Build history of the part. All positions in model axes, mm. Give positions to 0.01 mm unless a question says otherwise; leave off trailing zeros. Write each loop counter-clockwise with the first axis right and the second up, starting at its lowest first coordinate (ties: lowest second). Pieces come first, ordered by that corner, then holes.
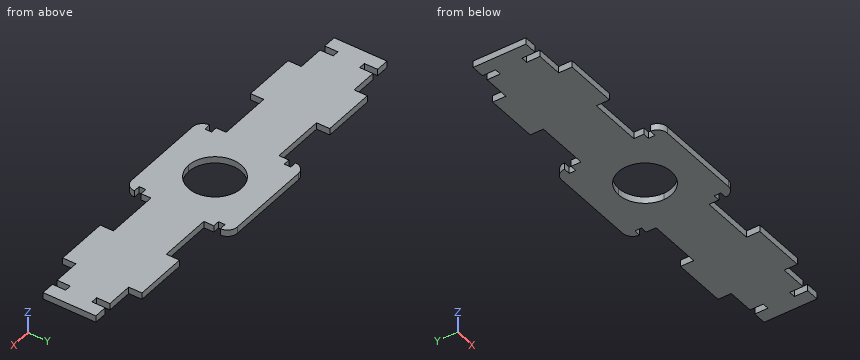
from build123d import *

# Parameters (mm, degrees)
BOSS_EXTRUDE1_DEPTH = 3.175
CUT_EXTRUDE3_DEPTH  = 3.175


with BuildPart() as part:
    # Sketch2 → Boss-Extrude1 (new body)
    with BuildSketch(Plane.XY):
        with BuildLine():
            Line((0, 12.7), (0, 25.4))
            Line((0, 25.4), (-98.425, 25.4))
            Line((-98.425, 25.4), (-98.425, -25.4))
            Line((-98.425, -25.4), (0, -25.4))
            Line((0, -25.4), (0, -12.7))
            ThreePointArc((0, -12.7), (-12.7, 0), (0, 12.7))
        make_face()
        with BuildLine():
            Line((98.425, 25.4), (0, 25.4))
            Line((0, 25.4), (0, 12.7))
            ThreePointArc((0, 12.7), (8.980256121, 8.980256121), (12.7, 0))
            ThreePointArc((12.7, 0), (8.980256121, -8.980256121), (0, -12.7))
            Line((0, -12.7), (0, -25.4))
            Line((0, -25.4), (98.425, -25.4))
            Line((98.425, -25.4), (98.425, 25.4))
        make_face()
    extrude(amount=BOSS_EXTRUDE1_DEPTH)

    # Sketch6 → Cut-Extrude3 (cut)
    with BuildSketch(Plane.XY):
        with BuildLine():
            Line((-22.225, 20.6375), (-25.4, 20.6375))
            ThreePointArc((-25.4, 20.6375), (-24.005096045, 24.005096045), (-20.6375, 25.4))
            Line((-20.6375, 25.4), (-25.4, 25.4))
            Line((-25.4, 25.4), (-98.425, 25.4))
            Line((-98.425, 25.4), (-98.425, 12.7))
            Line((-98.425, 12.7), (-92.075, 12.7))
            Line((-92.075, 12.7), (-92.075, 6.35))
            Line((-92.075, 6.35), (-88.9, 6.35))
            Line((-88.9, 6.35), (-88.9, 12.7))
            Line((-88.9, 12.7), (-76.2, 12.7))
            Line((-76.2, 12.7), (-76.2, 19.05))
            Line((-76.2, 19.05), (-50.8, 19.05))
            Line((-50.8, 19.05), (-50.8, 12.7))
            Line((-50.8, 12.7), (-25.4, 12.7))
            Line((-25.4, 12.7), (-25.4, 17.4625))
            Line((-25.4, 17.4625), (-22.225, 17.4625))
            Line((-22.225, 17.4625), (-22.225, 20.6375))
        make_face()
        with BuildLine():
            ThreePointArc((25.4, 20.6375), (24.005096045, 24.005096045), (20.6375, 25.4))
            Line((20.6375, 25.4), (25.4, 25.4))
            Line((25.4, 25.4), (98.425, 25.4))
            Line((98.425, 25.4), (98.425, 12.7))
            Line((98.425, 12.7), (92.075, 12.7))
            Line((92.075, 12.7), (92.075, 6.35))
            Line((92.075, 6.35), (88.9, 6.35))
            Line((88.9, 6.35), (88.9, 12.7))
            Line((88.9, 12.7), (76.2, 12.7))
            Line((76.2, 12.7), (76.2, 19.05))
            Line((76.2, 19.05), (50.8, 19.05))
            Line((50.8, 19.05), (50.8, 12.7))
            Line((50.8, 12.7), (25.4, 12.7))
            Line((25.4, 12.7), (25.4, 17.4625))
            Line((25.4, 17.4625), (22.225, 17.4625))
            Line((22.225, 17.4625), (22.225, 20.6375))
            Line((22.225, 20.6375), (25.4, 20.6375))
        make_face()
        with BuildLine():
            ThreePointArc((-25.4, -20.6375), (-24.005096045, -24.005096045), (-20.6375, -25.4))
            Line((-20.6375, -25.4), (-25.4, -25.4))
            Line((-25.4, -25.4), (-98.425, -25.4))
            Line((-98.425, -25.4), (-98.425, -12.7))
            Line((-98.425, -12.7), (-92.075, -12.7))
            Line((-92.075, -12.7), (-92.075, -6.35))
            Line((-92.075, -6.35), (-88.9, -6.35))
            Line((-88.9, -6.35), (-88.9, -12.7))
            Line((-88.9, -12.7), (-76.2, -12.7))
            Line((-76.2, -12.7), (-76.2, -19.05))
            Line((-76.2, -19.05), (-50.8, -19.05))
            Line((-50.8, -19.05), (-50.8, -12.7))
            Line((-50.8, -12.7), (-25.4, -12.7))
            Line((-25.4, -12.7), (-25.4, -17.4625))
            Line((-25.4, -17.4625), (-22.225, -17.4625))
            Line((-22.225, -17.4625), (-22.225, -20.6375))
            Line((-22.225, -20.6375), (-25.4, -20.6375))
        make_face()
        with BuildLine():
            Line((22.225, -20.6375), (25.4, -20.6375))
            ThreePointArc((25.4, -20.6375), (24.005096045, -24.005096045), (20.6375, -25.4))
            Line((20.6375, -25.4), (25.4, -25.4))
            Line((25.4, -25.4), (98.425, -25.4))
            Line((98.425, -25.4), (98.425, -12.7))
            Line((98.425, -12.7), (92.075, -12.7))
            Line((92.075, -12.7), (92.075, -6.35))
            Line((92.075, -6.35), (88.9, -6.35))
            Line((88.9, -6.35), (88.9, -12.7))
            Line((88.9, -12.7), (76.2, -12.7))
            Line((76.2, -12.7), (76.2, -19.05))
            Line((76.2, -19.05), (50.8, -19.05))
            Line((50.8, -19.05), (50.8, -12.7))
            Line((50.8, -12.7), (25.4, -12.7))
            Line((25.4, -12.7), (25.4, -17.4625))
            Line((25.4, -17.4625), (22.225, -17.4625))
            Line((22.225, -17.4625), (22.225, -20.6375))
        make_face()
    extrude(amount=CUT_EXTRUDE3_DEPTH, mode=Mode.SUBTRACT)


solid = part.part
(1) Saw through at D-D, the plane x = -69. List the corners of the cut face in (y, z) (3 decimals), plus the area to 3 significant figures.
(2) Saw through at A-A, the plane x = 2.5. List the corners of the cut face in (y, z) (1 decimal).
(3) Drop flat-ended pins along their axis: pin 1 (1.6 mm diameter, centred on x = -94.5, z = 1, fed in from -Y); pin 2 (1.6 mm diameter, centred on x = -95, z = 2, fed in from +Y); pin 3 (1.6 mm diameter, centred on y = 15, z = 2.5, fed in from +X). Give the stop position or say it passes through.
(4) Saw through at C-C, the plane y = -9. List the corners of the cut face in (x, z) (3 decimals), plus the area to 3 significant figures.
(5) Saw through at B-B, the plane y = 2. List the corners of the cut face in (x, z) (3 decimals).
(6) Probe line 1 (X direction, y = 9.5, z = 0.6) (3 decimals); line 2 (X direction, y = -14.5, z = 1.65); line 3 (X direction, y = 8.5, z = 0.9) (3 decimals). List the from-to ranges inside material, lowest first.
Computed values:
1. outline: (-19.05, 0) - (19.05, 0) - (19.05, 3.175) - (-19.05, 3.175) - close
1. area: 121 mm2
2. outline: (-25.4, 0) - (-12.5, 0) - (-12.5, 3.2) - (-25.4, 3.2) - close; (12.5, 0) - (25.4, 0) - (25.4, 3.2) - (12.5, 3.2) - close
3. pin 1: stops at y = -12.7
3. pin 2: stops at y = 12.7
3. pin 3: stops at x = 76.2
4. outline: (-98.425, 0) - (-92.075, 0) - (-92.075, 3.175) - (-98.425, 3.175) - close; (-88.9, 0) - (-8.96, 0) - (-8.96, 3.175) - (-88.9, 3.175) - close; (8.96, 0) - (88.9, 0) - (88.9, 3.175) - (8.96, 3.175) - close; (92.075, 0) - (98.425, 0) - (98.425, 3.175) - (92.075, 3.175) - close
4. area: 548 mm2
5. outline: (-98.425, 0) - (-12.542, 0) - (-12.542, 3.175) - (-98.425, 3.175) - close; (12.542, 0) - (98.425, 0) - (98.425, 3.175) - (12.542, 3.175) - close
6. line 1: x = -98.425 to -92.075, -88.9 to -8.429, 8.429 to 88.9, 92.075 to 98.425
6. line 2: x = -76.2 to -50.8, -25.4 to 25.4, 50.8 to 76.2
6. line 3: x = -98.425 to -92.075, -88.9 to -9.436, 9.436 to 88.9, 92.075 to 98.425
